Answer from the drawing. Dimensions are ordinates in mm from the lowest x, y and z of the part. A direction names the side the tool comes from. Coordinates: 2 decimals unless noted, no trailing zeros. Write each loop counter-clockwise with the first axis right and the second up, starting at its lowest first coordinate (ties: lowest second). Pieces come first, ordered by that corner, then holes.
(1) Section D-D on z = 6 is taken. Write down the section's boundary in (x, y).
(2) Which of the six approach directions +Z, -Z, +X, -X, +Y, -Y give full straight-line access (tool end or side, diameter ignored) to the marked faces 4 and 5?
(3) Section A-A on y = 12 is taken. Write down the section's boundary in (x, z).
(4) Given pin 1 (3.5 mm diameter, centred on x = 12, y = 12, fed in from +Z); pin 2 (4 mm diameter, centred on x = 9.5, z = 5, fed in from +Y); pin 3 (2 mm diameter, centred on y = 8, z = 5, fed in from -X), each flat-ended and moving along its own axis, determine where each tip first touches the part or whether it passes through.
(5) Section C-C on z = 2.5 is taken. Write down the section's boundary in (x, y), then the cut area to 3 significant figures.
(6) Find the intervals of material crossed by probe 1 along Y at (x, z) = (12, 2.25); probe 2 along Y at (x, z) = (12, 3.25); probe 3 along X at (y, z) = (12, 4.5), in increasing order.
(7) The mould has two halves that part along X. Classify the marked faces 1, 2 and 3: +X half, -X half, draft (parallel to the pull), parting line (faces both ways), or undercut.
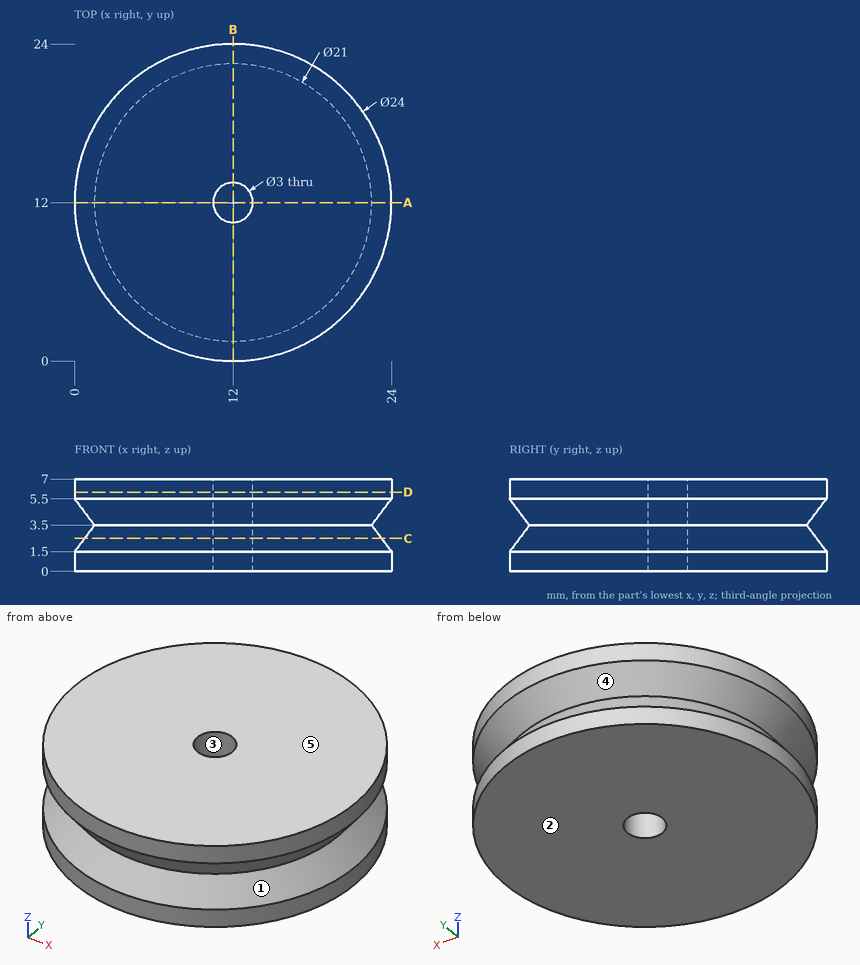
Response:
1. outline: circle Ø24 at (12, 12); hole circle Ø3 at (12, 12)
2. face 4: none
2. face 5: +Z, +X, -X, +Y, -Y
3. outline: (0, 0) - (10.5, 0) - (10.5, 7) - (0, 7) - (0, 5.5) - (1.5, 3.5) - (0, 1.5) - close; (13.5, 0) - (24, 0) - (24, 1.5) - (22.5, 3.5) - (24, 5.5) - (24, 7) - (13.5, 7) - close
4. pin 1: stops at z = 7
4. pin 2: stops at y = 23.99
4. pin 3: stops at x = 0.42
5. outline: circle Ø22.5 at (12, 12); hole circle Ø3 at (12, 12)
5. area: 391 mm2
6. probe 1: y = 0.56 to 10.5, 13.5 to 23.44
6. probe 2: y = 1.31 to 10.5, 13.5 to 22.69
6. probe 3: x = 0.75 to 10.5, 13.5 to 23.25
7. face 1: parting line
7. face 2: draft
7. face 3: undercut
